Work out the finished part from the listing and answer in its coordinate system (mm). Face numbers are marked on the shaded views. A direction names the side the tool comes from. Round coordinates to 2 decimals unless told otherwise and drop trailing zeros. Write each loop counter-clockwise with the first axis right and the second up, starting at its lowest first coordinate (ties: lowest second). Pieces come first, ordered by that corner, then holes. Notation, with made-up numbers: (71.5, -38.5) - (103.5, -38.5) arc R11 ccw to (103.5, -21.5) - close; hole circle Ø10 at (42.5, -39.5). An arc over 180 degrees is marked (long way). Answer as a JSON object with one key per item and string values.
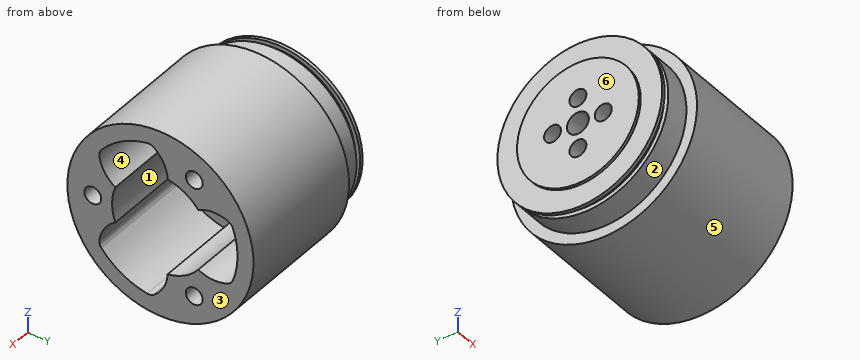
```python
from build123d import *

# Parameters (mm, degrees)
SKETCH4_R                  = 34.925
SKETCH4_R_2                = 18.161
BOSS_EXTRUDE1_DEPTH        = 72.771
CUT_EXTRUDE2_REACH         = 137.172
CUT_EXTRUDE2_START         = 21.75002
TRIPOD_WALLS_R             = 3.175
SKETCH12_R                 = 3.175
CUT_EXTRUDE3_DEPTH         = 63.5
CUT_EXTRUDE4_START         = -22.44598
SKETCH13_R                 = 34.925
CUT_EXTRUDE4_DEPTH         = 22.44598
SKETCH16_R                 = 22.86
COMPENSATING_SPACING_DEPTH = 1.016
F_1_4_0_2500_DOWEL_HOLE1_D = 6.35
BOLT_CIRCLE_PATTERN_2_R    = 4.1021
F_5_16_CLEARNCE_DEPTH      = 13.716


with BuildPart() as part:
    # Sketch2 → Revolve1 (revolve)
    with BuildSketch(Plane.XY, mode=Mode.PRIVATE) as revolve1_sk:
        Polygon((0, 0), (0, -30.9499), (12.7, -30.9499), (12.7, 0), (3.2004, 0), (3.2004, -1.5621), (1.27, -1.5621), (1.27, 0), align=None)
    revolve(revolve1_sk.sketch.rotate(Axis((11.964521893, -30.9499, 0), (-1, 0, 0)), 90), axis=Axis((11.964521893, -30.9499, 0), (-1, 0, 0)))

    # Sketch4 → Boss-Extrude1 (add)
    with BuildSketch(Plane(origin=(12.7, 0, 0), x_dir=(0, 0, -1), z_dir=(1, 0, 0))):
        with Locations((0, -30.9499)):
            Circle(SKETCH4_R)
        with Locations((0, -30.9499)):
            Circle(SKETCH4_R_2, mode=Mode.SUBTRACT)
    extrude(amount=BOSS_EXTRUDE1_DEPTH)

    # Sketch5 → Cut-Extrude2 (cut, up to next)
    with BuildSketch(Plane(origin=(0, 0, 0), x_dir=(0, 0, -1), z_dir=(1, 0, 0)).offset(CUT_EXTRUDE2_START), mode=Mode.PRIVATE) as cut_extrude2_sk1:
        with BuildLine():
            ThreePointArc((-11.141810341, -4.2233215), (0, -23.4823), (11.141810341, -4.2233215))
            ThreePointArc((11.141810341, -4.2233215), (0, -1.9939), (-11.141810341, -4.2233215))
        make_face()
    cut_extrude2_tool1 = extrude(cut_extrude2_sk1.sketch, amount=CUT_EXTRUDE2_REACH, mode=Mode.PRIVATE) & part.part
    # Sketch5 → Cut-Extrude2 (cut, up to next)
    with BuildSketch(Plane(origin=(0, 0, 0), x_dir=(0, 0, -1), z_dir=(1, 0, 0)).offset(CUT_EXTRUDE2_START), mode=Mode.PRIVATE) as cut_extrude2_sk2:
        with BuildLine():
            ThreePointArc((-28.716801071, -34.664098733), (-25.076631449, -45.427900247), (-17.57499054, -53.962280223))
            ThreePointArc((-17.57499054, -53.962280223), (-6.467131268, -34.683700064), (-28.716801071, -34.664098733))
        make_face()
    cut_extrude2_tool2 = extrude(cut_extrude2_sk2.sketch, amount=CUT_EXTRUDE2_REACH, mode=Mode.PRIVATE) & part.part
    # Sketch5 → Cut-Extrude2 (cut, up to next)
    with BuildSketch(Plane(origin=(0, 0, 0), x_dir=(0, 0, -1), z_dir=(1, 0, 0)).offset(CUT_EXTRUDE2_START), mode=Mode.PRIVATE) as cut_extrude2_sk3:
        with BuildLine():
            ThreePointArc((28.716801071, -34.664098733), (6.467131268, -34.683700064), (17.57499054, -53.962280223))
            ThreePointArc((17.57499054, -53.962280223), (25.076631449, -45.427900247), (28.716801071, -34.664098733))
        make_face()
    cut_extrude2_tool3 = extrude(cut_extrude2_sk3.sketch, amount=CUT_EXTRUDE2_REACH, mode=Mode.PRIVATE) & part.part
    add(cut_extrude2_tool1.solids().sort_by_distance((21.75002, -12.135894, 0))[0], mode=Mode.SUBTRACT)
    add(cut_extrude2_tool2.solids().sort_by_distance((21.75002, -40.356903, 16.293407))[0], mode=Mode.SUBTRACT)
    add(cut_extrude2_tool3.solids().sort_by_distance((21.75002, -40.356903, -16.293407))[0], mode=Mode.SUBTRACT)

    # Tripod walls
    tripod_walls_edges = [part.edges().sort_by_distance(p)[0] for p in [
        (53.61051, -4.2233215, 11.141810341),
        (53.61051, -4.2233215, -11.141810341),
        (53.61051, -53.962280223, 17.57499054),
        (53.61051, -34.664098733, 28.716801071),
        (53.61051, -34.664098733, -28.716801071),
        (53.61051, -53.962280223, -17.57499054),
    ]]
    fillet(tripod_walls_edges, radius=TRIPOD_WALLS_R)

    # Sketch12 → Cut-Extrude3 (cut)
    with BuildSketch(Plane(origin=(85.471, 0, 0), x_dir=(0, 0, -1), z_dir=(1, 0, 0))):
        with Locations((-21.997045256, -18.2499)):
            Circle(SKETCH12_R)
        with Locations((21.997045256, -18.2499)):
            Circle(SKETCH12_R)
        with Locations((0, -56.3499)):
            Circle(SKETCH12_R)
    extrude(amount=-CUT_EXTRUDE3_DEPTH, mode=Mode.SUBTRACT)

    # Sketch13 → Cut-Extrude4 (cut)
    with BuildSketch(Plane(origin=(85.471, 0, 0), x_dir=(0, 0, -1), z_dir=(1, 0, 0)).offset(CUT_EXTRUDE4_START)):
        with Locations((0, -30.9499)):
            Circle(SKETCH13_R)
    extrude(amount=CUT_EXTRUDE4_DEPTH, mode=Mode.SUBTRACT)

    # Sketch16 → Compensating Spacing (add)
    with BuildSketch(Plane.ZY):
        with Locations(Location((0, -30.9499, 0), (0, 0, 270))):
            Circle(SKETCH16_R)
    extrude(amount=COMPENSATING_SPACING_DEPTH)

    # 1/4 (0.2500) Dowel Hole1 (through all)
    with Locations(Plane(origin=(12.7, 0, 0), x_dir=(0, 0, -1), z_dir=(1, 0, 0))):
        with Locations((0, -21.4249), (9.525, -30.9499), (0, -40.4749), (-9.525, -30.9499)):
            Hole(F_1_4_0_2500_DOWEL_HOLE1_D / 2)

    # Bolt Circle Pattern<2> → 5/16 Clearnce (cut)
    with BuildSketch(Plane(origin=(12.7, 0, 0), x_dir=(0, 0, -1), z_dir=(1, 0, 0))):
        with Locations((0, -30.9499)):
            Circle(BOLT_CIRCLE_PATTERN_2_R)
    extrude(amount=-F_5_16_CLEARNCE_DEPTH, mode=Mode.SUBTRACT)


solid = part.part
```
Item 1: Determine the mould class of the marked faces 4, 5 and 6 for opening direction Y: pulls with the +Y half, pulls with the -Y half, needs draft (parallel to the pull), parting line crosses it, or undercut.
Results found:
{"face 4": "undercut", "face 5": "parting line crosses it", "face 6": "needs draft"}
Item 2: A cutting plane is placed at B-B (y = -22.5). Write down the section's boundary in (x, z), and give its area (3 significant figures).
Results found:
{"outline": "(-1.02, -21.24) - (0, -21.24) - (0, -29.77) - (1.27, -29.77) - (1.27, -28.15) - (3.2, -28.15) - (3.2, -29.77) - (12.7, -29.77) - (12.7, -33.89) - (63.03, -33.89) - (63.03, -16.08) - (12.7, -16.08) - (12.7, -2.99) - (-1.02, -2.99) - close; (-1.02, 2.99) - (12.7, 2.99) - (12.7, 16.08) - (63.03, 16.08) - (63.03, 33.89) - (12.7, 33.89) - (12.7, 29.77) - (3.2, 29.77) - (3.2, 28.15) - (1.27, 28.15) - (1.27, 29.77) - (0, 29.77) - (0, 21.24) - (-1.02, 21.24) - close", "area": "2,500 mm²"}
Item 3: Each of these flat-tipped pins is pushed along its axis until it touches: P1, Ø3, axis at y = -18.5, z = 22, coming from the +X side; P2, Ø10, axis at x = 8, y = -51.5, coming from the +Z side; P3, Ø8, axis at y = -9.5, z = -19, coming from the -X side; P4, Ø2, axis at y = -22, z = -2, coming from the +X side. Where does it stop, or does it pass through?
Results found:
{"P1": "x = 21.97", "P2": "z = 29.4", "P3": "x = 0", "P4": "through"}
Item 4: For the marked faces 1, 2 and 3, determine the directions among +Z, -Z, +X, -X, +Y, -Y from which every point of the face is accessible in a straight line to the end or side of a thin tool.
Results found:
{"face 1": "+X", "face 2": "-X", "face 3": "+Z, -Z, +X, +Y, -Y"}
Item 5: A cutting plane is placed at D-D (z = -14). Write down the section's boundary in (x, y).
Results found:
{"outline": "(-1.02, -49.02) - (0, -49.02) - (0, -58.55) - (1.27, -58.55) - (1.27, -56.79) - (3.2, -56.79) - (3.2, -58.55) - (12.7, -58.55) - (12.7, -62.95) - (63.03, -62.95) - (63.03, -53.45) - (21.75, -53.45) - (21.75, -42.52) - (12.7, -42.52) - (12.7, -19.38) - (63.03, -19.38) - (63.03, 1.05) - (12.7, 1.05) - (12.7, -3.35) - (3.2, -3.35) - (3.2, -5.11) - (1.27, -5.11) - (1.27, -3.35) - (0, -3.35) - (0, -12.88) - (-1.02, -12.88) - close"}
Item 6: Consider line 1 along Y through (x, z) = (9.75, 0); line 2 along Y through (x, z) = (60.5, 2); line 3 along Z through (x, y) = (26.5, -17). Determine where each line is inside the solid, lowest interval first.
Results found:
{"line 1": "-61.9 to -43.65, -37.3 to -35.05, -26.85 to -24.6, -18.25 to 0", "line 2": "-65.82 to -58.82, -53.88 to -49, -2.06 to 3.92", "line 3": "-32.02 to -24.92, -19.08 to -11.63, 11.63 to 19.08, 24.92 to 32.02"}
Item 7: A cutting plane is placed at C-C (x = 6). Write down the section's boundary in (y, z) (3 decimals).
Results found:
{"outline": "circle Ø61.9 at (-30.95, 0); hole circle Ø6.35 at (-40.475, 0); hole circle Ø8.204 at (-30.95, 0); hole circle Ø6.35 at (-30.95, -9.525); hole circle Ø6.35 at (-30.95, 9.525); hole circle Ø6.35 at (-21.425, 0)"}
Item 8: A cutting plane is placed at A-A (z = 0). Give the number of separate pieces and of enclosed holes in the cut face, and give its area (3 significant figures).
Results found:
{"separate pieces": "4", "enclosed holes": "0", "area": "1,520 mm²"}
